Verification items for the finished model (mm, model axes). A direction names the side the tool comes from. Round coordinates to 2 decimals unless told otherwise and drop trailing zeros. Order: outer loops, then holes, each group sorted by start corner. A loop starts at its lowest first (then second) coordinate and runs counter-clockwise, first axis right, second up. Notation, with made-up numbers: M -35,-13.5 L -15,-13.5 A16 cw -15,17.5 Z; hole C 88,87.25 d8. An arc over 180 degrees is marked long. Use one line per item in the form item = value. Start each with the question number.
Item 1: Go/stop test with flat-tipped pins: pin 1 Ø1.5 at (y, z) = (3.5, 1.5) entering from -X; pin 2 Ø1.5 at (x, z) = (-0.5, 0) entering from +Y; pin 3 Ø6 at (x, y) = (-2, -6.5) entering from -Z. Record where each tip stops, or that it passes through.
Item 2: Cross-section at A-A on y = 3.75. Enter the section's corners in (x, z).
Item 3: Cross-section at D-D on y = -5.25. Enter the section's corners in (x, z).
Item 4: Cross-section at B-B on x = 0. Enter the section's corners in (y, z), then the cut area to 3 significant figures.
Item 5: Cross-section at C-C on z = 2. Enter the section's corners in (x, y), then the cut area to 3 significant figures.
Item 6: Thickness scan on probe 1 along Z at (x, y) = (0, 1.75); probe 2 along Y at (x, z) = (-2.5, 0); probe 3 along Y at (x, z) = (3.5, -1.75). Record the ranges inside material, lowest first. Write a range as [from, to].
Item 7: Tool access check on faces 1 (the flat face through (0, -16, 0)), 2 (the flat face through (2.2, 0, 2.2)), 3 (the flat face through (-2.21, 3.73, 1.25)). Record the directions out of +Z, -Z, +X, -X, +Y, -Y that give a thin tool (end or side, any length) a straight path to the whole face; none if there is none.
Item 8: Release check for a two-part mould opening along Z. For faces 4 (the flat face through (2, 5.82, 2)), 5 (the flat face through (2.19, 3.73, 1.29)), 6 (the flat face through (0, 1.59, 0)), 7 (the cylindrical face through (-1.08, 2.87, 4.88)) record: +Z half, -Z half, draft (parallel to the pull), parting line (faces both ways), or undercut.
from build123d import *

# Parameters (mm, degrees)
SKETCH1_R           = 5
BOSS_EXTRUDE1_DEPTH = 5.82
SKETCH2_R           = 2.92
BOSS_EXTRUDE2_DEPTH = 16
CUT_EXTRUDE1_DEPTH  = 4.23


with BuildPart() as part:
    # Sketch1 → Boss-Extrude1 (new body)
    with BuildSketch(Plane(origin=(0, 0, 0), x_dir=(1, 0, 0), z_dir=(0, 1, 0))):
        Circle(SKETCH1_R)
    extrude(amount=BOSS_EXTRUDE1_DEPTH)

    # Sketch2 → Boss-Extrude2 (add)
    with BuildSketch(Plane.XZ):
        Circle(SKETCH2_R)
    extrude(amount=BOSS_EXTRUDE2_DEPTH)

    # Sketch3 → Cut-Extrude1 (cut)
    with BuildSketch(Plane(origin=(0, 5.82, 0), x_dir=(1, 0, 0), z_dir=(0, 1, 0))):
        Polygon((2.932939367, 0), (1.466469684, 2.54), (-1.466469684, 2.54), (-2.932939367, 0), (-1.466469684, -2.54), (1.466469684, -2.54), align=None)
    extrude(amount=-CUT_EXTRUDE1_DEPTH, mode=Mode.SUBTRACT)


solid = part.part
Output values:
q1.pin_1 = -4.94
q1.pin_2 = 1.59
q1.pin_3 = -2.92
q2.outline = C 0,0 d10; hole M -2.93,0 L -1.47,-2.54 L 1.47,-2.54 L 2.93,0 L 1.47,2.54 L -1.47,2.54 Z
q3.outline = C 0,0 d5.84
q4.outline = M -16,-2.92 L 0,-2.92 L 0,-5 L 5.82,-5 L 5.82,-2.54 L 1.59,-2.54 L 1.59,2.54 L 5.82,2.54 L 5.82,5 L 0,5 L 0,2.92 L -16,2.92 Z
q4.area = 130 mm2
q5.outline = M -4.58,0 L -2.13,0 L -2.13,-16 L 2.13,-16 L 2.13,0 L 4.58,0 L 4.58,5.82 L 1.78,5.82 L 1.78,1.59 L -1.78,1.59 L -1.78,5.82 L -4.58,5.82 Z
q5.area = 106 mm2
q6.probe_1 = [-5, -2.54], [2.54, 5]
q6.probe_2 = [-16, 1.59]
q6.probe_3 = [0, 5.82]
q7.face_1 = +Z, -Z, +X, -X, -Y
q7.face_2 = -Y
q7.face_3 = +Y
q8.face_4 = draft
q8.face_5 = undercut
q8.face_6 = undercut
q8.face_7 = parting line
